Drawing for the job (mm, zero at the part's lowest x, y, z). A direction names the side the tool comes from. Round coordinates to 2 decimals unless told otherwise and drop trailing zeros. Write each loop counter-clockwise with the first axis right and the second up, starting at its lowest first coordinate (ties: lowest second). Pieces come first, ordered by that corner, then holes. Notation, with made-up numbers: M 55,69 L 91,69 A25 ccw 91,81 Z; hole C -15,82 d5. An arc over 180 degrees is marked long. Use a Markdown table: item, result.
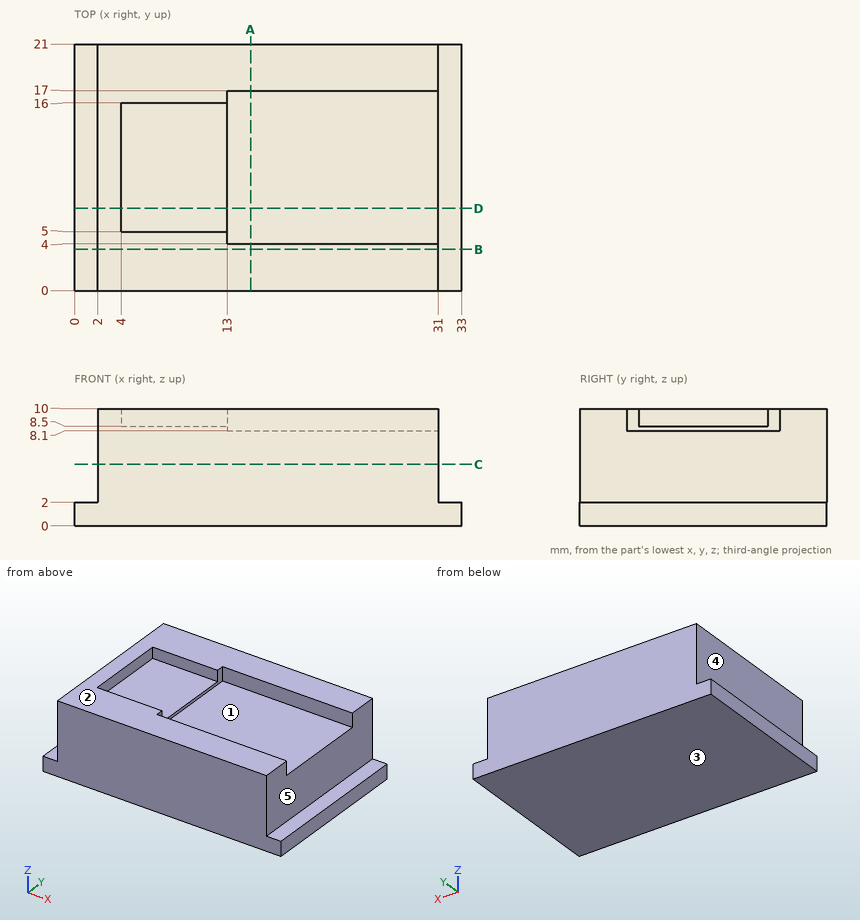
Q1. Cut at B-B on y = 3.5. Give the cut face in (x, z), and give its area (3 significant figures).
Response values:
| item | result |
|---|---|
| outline | M 0,0 L 33,0 L 33,2 L 31,2 L 31,10 L 2,10 L 2,2 L 0,2 Z |
| area | 298 mm2 |
Q2. Two-plate mould, pull along X, no slides. Class the marked faces 3, 4 and 5: +X half, -X half, draft (parallel to the pull), parting line (faces both ways), or undercut.
Response values:
| item | result |
|---|---|
| face 3 | draft |
| face 4 | -X half |
| face 5 | +X half |
Q3. Which spindle directions (+Z, -Z, +X, -X, +Y, -Y) get a long thin tool onto all of the face, cutting with end or side? Do the marked faces 1 and 2. Say none if no direction does.
Response values:
| item | result |
|---|---|
| face 1 | +Z, +X |
| face 2 | +Z, +X, -X, +Y, -Y |
Q4. Cut at D-D on y = 7. Give the cut face in (x, z), and give its area (3 significant figures).
Response values:
| item | result |
|---|---|
| outline | M 0,0 L 33,0 L 33,2 L 31,2 L 31,8.1 L 13,8.1 L 13,8.5 L 4,8.5 L 4,10 L 2,10 L 2,2 L 0,2 Z |
| area | 250 mm2 |
Q5. Cut at A-A on x = 15. Give the cut face in (y, z).
Response values:
| item | result |
|---|---|
| outline | M 0,0 L 21,0 L 21,10 L 17,10 L 17,8.1 L 4,8.1 L 4,10 L 0,10 Z |
Q6. Drop a flat-ended pin along its axis: P1, Ø0.6, axis at y = 9, z = 9, coming from the +X side. Give the stop position or say it passes through.
Response values:
| item | result |
|---|---|
| P1 | stops at x = 4 |
Q7. Drill centre lines: L1, parallel to X at y = 9, z = 5; L2, parallel to Z at x = 24.5, y = 13.25; L3, parallel to Z at x = 12, y = 14.25. Where is each one in solid material? Low to high.
Response values:
| item | result |
|---|---|
| L1 | x = 2 to 31 |
| L2 | z = 0 to 8.1 |
| L3 | z = 0 to 8.5 |
Q8. Cut at C-C on z = 5.25. Give the cut face in (x, y), and give its area (3 significant figures).
Response values:
| item | result |
|---|---|
| outline | M 2,0 L 31,0 L 31,21 L 2,21 Z |
| area | 609 mm2 |
